Answer from the drawing. Dimensions are ordinates in mm from the lowest x, y and z of the part. Coordinates: 2 decimals unless noted, no trailing zeros. Write each loop counter-clockwise with the first axis right and the second up, starting at its lowest first coordinate (ties: lowest second). Pieces come first, ordered by that corner, then holes.
(1) Given pin 1 (3 mm diameter, centred on x = 65.5, y = 4, fed in from +Z); pin 2 (1.9 mm diameter, centred on x = 66, y = 3.5, fed in from -Z), each flat-ended and moving along its own axis, determine where each tip first touches the part or whether it passes through.
(2) Find the intervals of material crossed by probe 1 along X at (y, z) = (2, 9.5); probe 2 along Z at (x, y) = (66.5, 2), in increasing order.
(3) Section B-B on x = 66 is taken. Write down the section's boundary in (y, z), then the cut area to 3 significant figures.
(4) Section A-A on y = 2.75 is taken. Write down the section's boundary in (x, z).
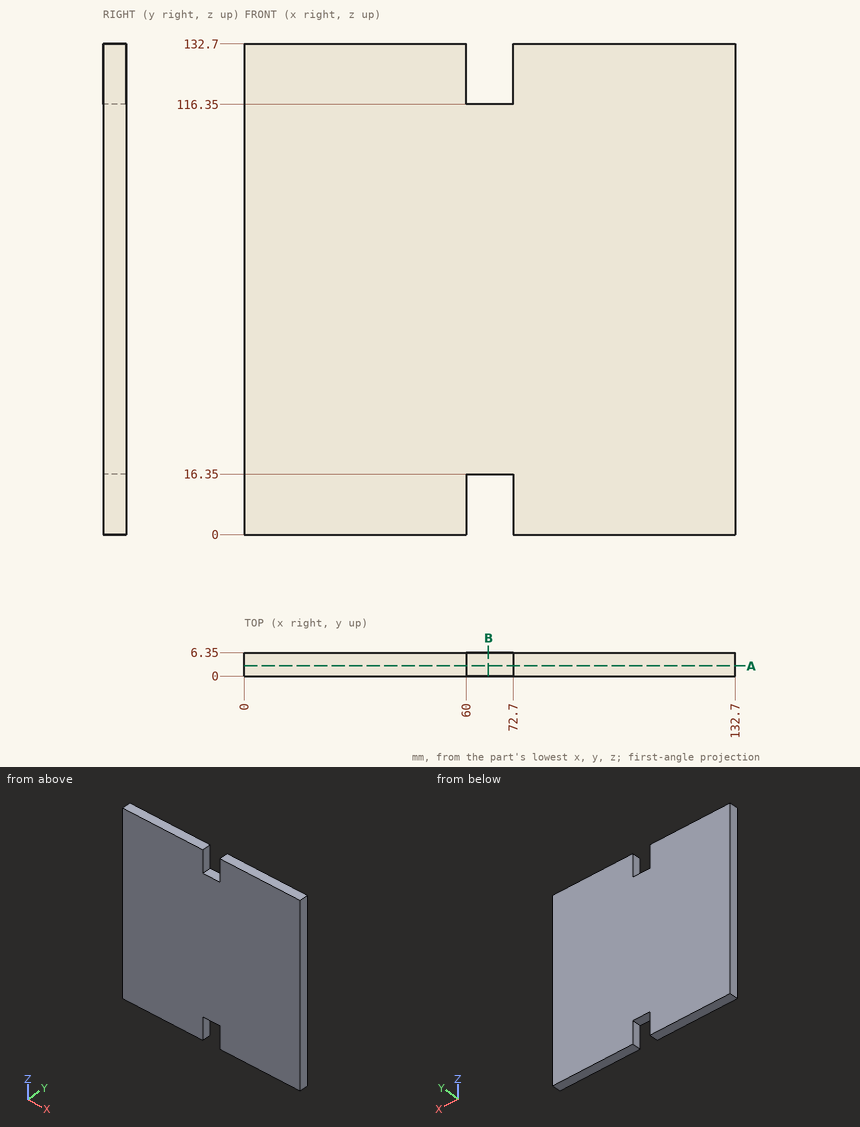
Response:
1. pin 1: stops at z = 116.35
1. pin 2: stops at z = 16.35
2. probe 1: x = 0 to 60, 72.7 to 132.7
2. probe 2: z = 16.35 to 116.35
3. outline: (0, 16.35) - (6.35, 16.35) - (6.35, 116.35) - (0, 116.35) - close
3. area: 635 mm2
4. outline: (0, 0) - (60, 0) - (60, 16.35) - (72.7, 16.35) - (72.7, 0) - (132.7, 0) - (132.7, 132.7) - (72.7, 132.7) - (72.7, 116.35) - (60, 116.35) - (60, 132.7) - (0, 132.7) - close
